Check sheet for the drawn part. Datum: minimum x, y, z corner. Units: mm. A direction names the side the tool comes from. Coordinates: 2 decimals unless noted, no trailing zeros. Order: outer loops, then holes, each group sorted by start corner. A loop starts at its lowest first (then second) coordinate and runs counter-clockwise, first axis right, second up. Notation, with made-up numbers: M -8,52 L 51,52 A22 ccw 51,81 Z; hole C 70.25,-22 d7. An arc over 180 degrees is marked long. Return JSON: item names as keys, results as strings. Group by question number.
Q1. Section check C-C, the plane y = 16.5. Enter the section's corners in (x, z), then the cut area to 4 significant figures.
Q2. Go/stop test with flat-tipped pins: pin 1 Ø12 at (x, z) = (40.5, 25.5) entering from +Y; pin 2 Ø2.5 at (y, z) = (10, 37.5) entering from -X. Record where each tip stops, or that it passes through.
Q3. Mould release check, pull along X, two halves, no side actions. Record for the marked faces 1, 2 and 3: pulls with the +X half, pulls with the -X half, needs draft (parallel to the pull), parting line crosses it, or undercut.
Q4. Thickness scan on probe 1 along Y at (x, z) = (50.1, 6.5); probe 2 along Y at (x, z) = (49.6, 22); probe 3 along X at (y, z) = (4.5, 39.5). Record the ranges inside material, lowest first.
Q5. Section check A-A, the plane y = 25.5. Enter the section's corners in (x, z).
Q6. Section check D-D, the plane z = 41.5. Enter the section's corners in (x, y).
Q7. Access from +Z, -Z, +X, -X, +Y, -Y to the whole of each face (thin tool, end or side, straight path). Record for the marked faces 4 and 5.
Q8. Section check B-B, the plane z = 22. Count the separate pieces of the cut face and the enclosed holes in it, then the cut area to 3 significant figures.
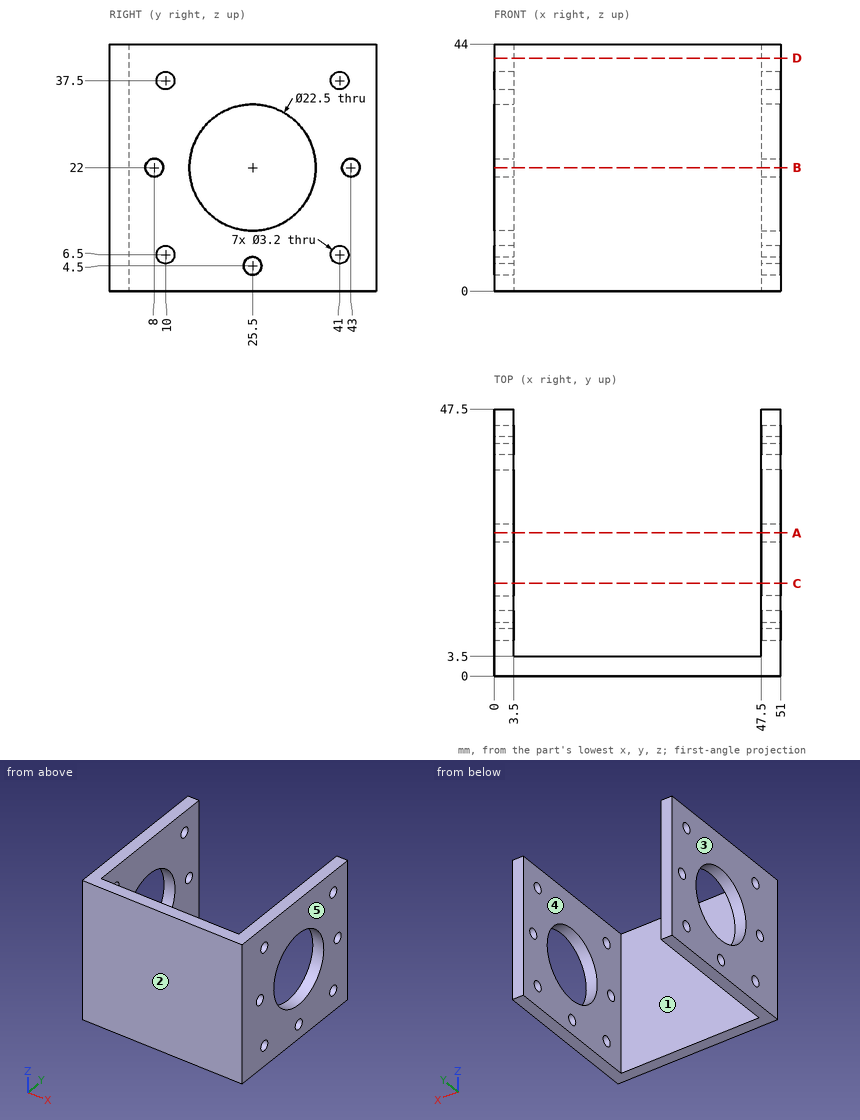
Numbers:
{
 "1": {"outline": "M 0,0 L 3.5,0 L 3.5,15.25 L 0,15.25 Z; M 0,28.75 L 3.5,28.75 L 3.5,44 L 0,44 Z; M 47.5,0 L 51,0 L 51,15.25 L 47.5,15.25 Z; M 47.5,28.75 L 51,28.75 L 51,44 L 47.5,44 Z", "area": "213.5 mm2"},
 "2": {"pin 1": "stops at y = 3.5", "pin 2": "passes through"},
 "3": {"face 1": "undercut", "face 2": "needs draft", "face 3": "pulls with the -X half"},
 "4": {"probe 1": "y = 0 to 8.4, 11.6 to 39.4, 42.6 to 47.5", "probe 2": "y = 0 to 6.4, 9.6 to 14.25, 36.75 to 41.4, 44.6 to 47.5", "probe 3": "x = 0 to 3.5, 47.5 to 51"},
 "5": {"outline": "M 0,0 L 3.5,0 L 3.5,2.9 L 0,2.9 Z; M 0,6.1 L 3.5,6.1 L 3.5,10.75 L 0,10.75 Z; M 0,33.25 L 3.5,33.25 L 3.5,44 L 0,44 Z; M 47.5,0 L 51,0 L 51,2.9 L 47.5,2.9 Z; M 47.5,6.1 L 51,6.1 L 51,10.75 L 47.5,10.75 Z; M 47.5,33.25 L 51,33.25 L 51,44 L 47.5,44 Z"},
 "6": {"outline": "M 0,0 L 51,0 L 51,47.5 L 47.5,47.5 L 47.5,3.5 L 3.5,3.5 L 3.5,47.5 L 0,47.5 Z"},
 "7": {"face 4": "+Z, -Z, +Y", "face 5": "+Z, -Z, +X, +Y, -Y"},
 "8": {"separate pieces": "7", "enclosed holes": "0", "area": "284 mm2"}
}
